Source: CAD feature listing. Evaluate the final solid. Frame: model axes, mm. A direction names the side the tool comes from. Coordinates: 2 decimals unless noted, no trailing zeros. Write each loop counter-clockwise with the first axis right and the second up, starting at its lowest first coordinate (ties: lowest second). Pieces come first, ordered by that corner, then holes. Notation, with made-up numbers: (69.5, -38) -> (97.5, -38) arc R25 cw to (97.5, 0) -> close; hole circle Ø5 at (73, -0.5). An arc over 180 degrees is marked (long way). Write item = value, one per line.
from build123d import *

# Parameters (mm, degrees)
SKETCH1_W           = 40.44093781
SKETCH1_H           = 22.193197578
BOSS_EXTRUDE1_DEPTH = 3.81
SKETCH3_R           = 3.4925
CUT_EXTRUDE3_DEPTH  = 2.794
SKETCH3_4_R         = 1.7018
CUT_EXTRUDE4_DEPTH  = 24.377723743


with BuildPart() as part:
    # Sketch1 → Boss-Extrude1 (new body)
    with BuildSketch(Plane(origin=(0, 0, 0), x_dir=(1, 0, 0), z_dir=(0, 1, 0))):
        Rectangle(SKETCH1_W, SKETCH1_H)
    extrude(amount=BOSS_EXTRUDE1_DEPTH)

    # Sketch3 → Cut-Extrude3 (cut)
    with BuildSketch(Plane(origin=(0, 3.81, 0), x_dir=(1, 0, 0), z_dir=(0, 1, 0))):
        with Locations(Location((-16.156468905, 7.032598789, 0), (0, 0, 270))):
            Circle(SKETCH3_R)
        with Locations(Location((16.156468905, -7.032598789, 0), (0, 0, 270))):
            Circle(SKETCH3_R)
    extrude(amount=-CUT_EXTRUDE3_DEPTH, mode=Mode.SUBTRACT)

    # Sketch3_4 → Cut-Extrude4 (cut, through all)
    with BuildSketch(Plane(origin=(0, 3.81, 0), x_dir=(1, 0, 0), z_dir=(0, 1, 0))):
        with Locations(Location((-16.156468905, 7.032598789, 0), (0, 0, 270))):
            Circle(SKETCH3_4_R)
        with Locations(Location((16.156468905, -7.032598789, 0), (0, 0, 270))):
            Circle(SKETCH3_4_R)
    extrude(amount=-CUT_EXTRUDE4_DEPTH, mode=Mode.SUBTRACT)


solid = part.part
1) Cut plane D-D, the plane z = 6. Output: boundary loops of the cut face in (x, y), and give its area (3 significant figures).
Answer block:
outline = (-20.22, 0) -> (14.8, 0) -> (14.8, 1.02) -> (12.82, 1.02) -> (12.82, 3.81) -> (-20.22, 3.81) -> close; (17.51, 0) -> (20.22, 0) -> (20.22, 3.81) -> (19.49, 3.81) -> (19.49, 1.02) -> (17.51, 1.02) -> close
area = 133 mm2
2) Pull-direction query (Z, two-part tool) for faces 1 (the flat face through (20.22, 2, 0)), 2 (the flat face through (-18, 1.016, -8)), 3 (the flat face through (0, 2, 11.097)), 4 (the flat face through (0, 2, -11.097)); classes: +Z half, -Z half, draft (parallel to the pull), parting line (faces both ways), or undercut.
Answer block:
face_1 = draft
face_2 = undercut
face_3 = +Z half
face_4 = -Z half
3) Reachability of faces 5 (the flat face through (0, 0, 0)), 6 (the cylindrical face through (12.747, 2.433, 6.275)) from +Z, -Z, +X, -X, +Y, -Y: full face, straight path, thin tool, end or side. Return the list, or none.
Answer block:
face_5 = +Z, -Z, +X, -X, -Y
face_6 = +Y
4) Material intervals for probe 1 along X at (y, z) = (2.05, 5.25); probe 2 along Z at (x, y) = (17, 0.4); probe 3 along X at (y, z) = (1.6, -9), sorted ascending. Write a range as [from, to].
Answer block:
probe_1 = [-20.22, 13.15], [19.16, 20.22]
probe_2 = [-11.1, 5.55], [8.51, 11.1]
probe_3 = [-20.22, -19.04], [-13.27, 20.22]
5) Cut plane A-A, the plane z = -6.5. Output: boundary loops of the cut face in (x, y).
Answer block:
outline = (-20.22, 0) -> (-17.77, 0) -> (-17.77, 1.02) -> (-19.61, 1.02) -> (-19.61, 3.81) -> (-20.22, 3.81) -> close; (-14.54, 0) -> (20.22, 0) -> (20.22, 3.81) -> (-12.7, 3.81) -> (-12.7, 1.02) -> (-14.54, 1.02) -> close
6) First-contact query: pin 1 Ø5.5 at (x, z) = (-16.16, -7.03) entering from +Y; pin 2 Ø8 at (x, z) = (-13, 4) entering from -Y; pin 3 Ø3 at (x, z) = (-16.16, -7.03) entering from +Y. Flat tips, straight axial feed; report the tip coordinate or a pass-through.
Answer block:
pin_1 = 1.02
pin_2 = 0
pin_3 = through
7) Cut plane C-C, the plane z = -4. Output: boundary loops of the cut face in (x, y).
Answer block:
outline = (-20.22, 0) -> (20.22, 0) -> (20.22, 3.81) -> (-14.42, 3.81) -> (-14.42, 1.02) -> (-17.89, 1.02) -> (-17.89, 3.81) -> (-20.22, 3.81) -> close
8) Cut plane B-B, the plane y = 0.6. Output: boundary loops of the cut face in (x, z).
Answer block:
outline = (-20.22, -11.1) -> (20.22, -11.1) -> (20.22, 11.1) -> (-20.22, 11.1) -> close; hole circle Ø3.4 at (-16.16, -7.03); hole circle Ø3.4 at (16.16, 7.03)
